from build123d import *

# Parameters (mm, degrees)
SKETCH2_W                     = 6.6
SKETCH2_H                     = 9.76
BOSS_EXTRUDE1_DEPTH           = 1.75
BOSS_EXTRUDE1_TAPER           = 15
BOSS_EXTRUDE1_OTHER_WAY_DEPTH = 1.75
BOSS_EXTRUDE1_OTHER_WAY_TAPER = 15
BOSS_EXTRUDE2_DEPTH           = 0.65
FILLET1_R                     = 0.15
BOSS_EXTRUDE3_DEPTH           = 0.65
BOSS_EXTRUDE4_DEPTH           = 0.65
BOSS_EXTRUDE5_DEPTH           = 0.65


with BuildPart() as part:
    # Sketch2 → Boss-Extrude1 (new body)
    with BuildSketch(Plane(origin=(0, 0, 0), x_dir=(1, 0, 0), z_dir=(0, 1, 0))):
        Rectangle(SKETCH2_W, SKETCH2_H)
    extrude(amount=BOSS_EXTRUDE1_DEPTH, taper=BOSS_EXTRUDE1_TAPER)

    # Sketch2 → Boss-Extrude1 other way (add)
    with BuildSketch(Plane(origin=(0, 0, 0), x_dir=(1, 0, 0), z_dir=(0, 1, 0))):
        Rectangle(SKETCH2_W, SKETCH2_H)
    extrude(amount=-BOSS_EXTRUDE1_OTHER_WAY_DEPTH, taper=BOSS_EXTRUDE1_OTHER_WAY_TAPER)

    # Sketch3 → Boss-Extrude2 (add, symmetric)
    with BuildSketch(Plane.XY.offset(3.66)):
        Polygon((3.266506351, 0.125), (3.3, 0), (3.266506351, -0.125), (3.616889449, -0.125), (4.25, -2.55), (5.15, -2.55), (5.15, -2.3), (4.443110551, -2.3), (3.81, 0.125), align=None)
        Polygon((-4.25, -2.55), (-5.15, -2.55), (-5.15, -2.3), (-4.443110551, -2.3), (-3.81, 0.125), (-3.266506351, 0.125), (-3.3, 0), (-3.266506351, -0.125), (-3.616889449, -0.125), align=None)
    extrude(amount=BOSS_EXTRUDE2_DEPTH, both=True)

    # Fillet1
    fillet1_edges = [part.edges().sort_by_distance(p)[0] for p in [
        (4.443110551, -2.3, 3.66),
        (3.81, 0.125, 3.66),
        (3.616889449, -0.125, 3.66),
        (4.25, -2.55, 3.66),
        (-4.25, -2.55, 3.66),
        (-3.616889449, -0.125, 3.66),
        (-3.81, 0.125, 3.66),
        (-4.443110551, -2.3, 3.66),
    ]]
    fillet(fillet1_edges, radius=FILLET1_R)

    # Sketch5 → Boss-Extrude3 (add, symmetric)
    with BuildSketch(Plane.XY.offset(1.22)):
        with BuildLine():
            Line((-5.15, -2.55), (-4.365866331, -2.55))
            ThreePointArc((-4.365866331, -2.55), (-4.274170395, -2.518709121), (-4.220731079, -2.437891406))
            Line((-4.220731079, -2.437891406), (-3.64615837, -0.237108594))
            ThreePointArc((-3.64615837, -0.237108594), (-3.592719053, -0.156290879), (-3.501023118, -0.125))
            Line((-3.501023118, -0.125), (-3.266506351, -0.125))
            Line((-3.266506351, -0.125), (-3.3, 0))
            Line((-3.3, 0), (-3.266506351, 0.125))
            Line((-3.266506351, 0.125), (-3.694133669, 0.125))
            ThreePointArc((-3.694133669, 0.125), (-3.785829605, 0.093709121), (-3.839268921, 0.012891406))
            Line((-3.839268921, 0.012891406), (-4.41384163, -2.187891406))
            ThreePointArc((-4.41384163, -2.187891406), (-4.467280947, -2.268709121), (-4.558976882, -2.3))
            Line((-4.558976882, -2.3), (-5.15, -2.3))
            Line((-5.15, -2.3), (-5.15, -2.55))
        make_face()
        with BuildLine():
            Line((3.64615837, -0.237108594), (4.220731079, -2.437891406))
            ThreePointArc((4.220731079, -2.437891406), (4.274170395, -2.518709121), (4.365866331, -2.55))
            Line((4.365866331, -2.55), (5.15, -2.55))
            Line((5.15, -2.55), (5.15, -2.3))
            Line((5.15, -2.3), (4.558976882, -2.3))
            ThreePointArc((4.558976882, -2.3), (4.467280947, -2.268709121), (4.41384163, -2.187891406))
            Line((4.41384163, -2.187891406), (3.839268921, 0.012891406))
            ThreePointArc((3.839268921, 0.012891406), (3.785829605, 0.093709121), (3.694133669, 0.125))
            Line((3.694133669, 0.125), (3.266506351, 0.125))
            Line((3.266506351, 0.125), (3.3, 0))
            Line((3.3, 0), (3.266506351, -0.125))
            Line((3.266506351, -0.125), (3.501023118, -0.125))
            ThreePointArc((3.501023118, -0.125), (3.592719053, -0.156290879), (3.64615837, -0.237108594))
        make_face()
    extrude(amount=BOSS_EXTRUDE3_DEPTH, both=True)

    # Sketch6 → Boss-Extrude4 (add, symmetric)
    with BuildSketch(Plane.XY.offset(-1.22)):
        with BuildLine():
            Line((3.64615837, -0.237108594), (4.220731079, -2.437891406))
            ThreePointArc((4.220731079, -2.437891406), (4.274170395, -2.518709121), (4.365866331, -2.55))
            Line((4.365866331, -2.55), (5.15, -2.55))
            Line((5.15, -2.55), (5.15, -2.3))
            Line((5.15, -2.3), (4.558976882, -2.3))
            ThreePointArc((4.558976882, -2.3), (4.467280947, -2.268709121), (4.41384163, -2.187891406))
            Line((4.41384163, -2.187891406), (3.839268921, 0.012891406))
            ThreePointArc((3.839268921, 0.012891406), (3.785829605, 0.093709121), (3.694133669, 0.125))
            Line((3.694133669, 0.125), (3.266506351, 0.125))
            Line((3.266506351, 0.125), (3.3, 0))
            Line((3.3, 0), (3.266506351, -0.125))
            Line((3.266506351, -0.125), (3.501023118, -0.125))
            ThreePointArc((3.501023118, -0.125), (3.592719053, -0.156290879), (3.64615837, -0.237108594))
        make_face()
        with BuildLine():
            Line((-5.15, -2.55), (-4.365866331, -2.55))
            ThreePointArc((-4.365866331, -2.55), (-4.274170395, -2.518709121), (-4.220731079, -2.437891406))
            Line((-4.220731079, -2.437891406), (-3.64615837, -0.237108594))
            ThreePointArc((-3.64615837, -0.237108594), (-3.592719053, -0.156290879), (-3.501023118, -0.125))
            Line((-3.501023118, -0.125), (-3.266506351, -0.125))
            Line((-3.266506351, -0.125), (-3.3, 0))
            Line((-3.3, 0), (-3.266506351, 0.125))
            Line((-3.266506351, 0.125), (-3.694133669, 0.125))
            ThreePointArc((-3.694133669, 0.125), (-3.785829605, 0.093709121), (-3.839268921, 0.012891406))
            Line((-3.839268921, 0.012891406), (-4.41384163, -2.187891406))
            ThreePointArc((-4.41384163, -2.187891406), (-4.467280947, -2.268709121), (-4.558976882, -2.3))
            Line((-4.558976882, -2.3), (-5.15, -2.3))
            Line((-5.15, -2.3), (-5.15, -2.55))
        make_face()
    extrude(amount=BOSS_EXTRUDE4_DEPTH, both=True)

    # Sketch7 → Boss-Extrude5 (add, symmetric)
    with BuildSketch(Plane.XY.offset(-3.66)):
        with BuildLine():
            Line((3.64615837, -0.237108594), (4.220731079, -2.437891406))
            ThreePointArc((4.220731079, -2.437891406), (4.274170395, -2.518709121), (4.365866331, -2.55))
            Line((4.365866331, -2.55), (5.15, -2.55))
            Line((5.15, -2.55), (5.15, -2.3))
            Line((5.15, -2.3), (4.558976882, -2.3))
            ThreePointArc((4.558976882, -2.3), (4.467280947, -2.268709121), (4.41384163, -2.187891406))
            Line((4.41384163, -2.187891406), (3.839268921, 0.012891406))
            ThreePointArc((3.839268921, 0.012891406), (3.785829605, 0.093709121), (3.694133669, 0.125))
            Line((3.694133669, 0.125), (3.266506351, 0.125))
            Line((3.266506351, 0.125), (3.3, 0))
            Line((3.3, 0), (3.266506351, -0.125))
            Line((3.266506351, -0.125), (3.501023118, -0.125))
            ThreePointArc((3.501023118, -0.125), (3.592719053, -0.156290879), (3.64615837, -0.237108594))
        make_face()
        with BuildLine():
            Line((-5.15, -2.3), (-5.15, -2.55))
            Line((-5.15, -2.55), (-4.365866331, -2.55))
            ThreePointArc((-4.365866331, -2.55), (-4.274170395, -2.518709121), (-4.220731079, -2.437891406))
            Line((-4.220731079, -2.437891406), (-3.64615837, -0.237108594))
            ThreePointArc((-3.64615837, -0.237108594), (-3.592719053, -0.156290879), (-3.501023118, -0.125))
            Line((-3.501023118, -0.125), (-3.266506351, -0.125))
            Line((-3.266506351, -0.125), (-3.3, 0))
            Line((-3.3, 0), (-3.266506351, 0.125))
            Line((-3.266506351, 0.125), (-3.694133669, 0.125))
            ThreePointArc((-3.694133669, 0.125), (-3.785829605, 0.093709121), (-3.839268921, 0.012891406))
            Line((-3.839268921, 0.012891406), (-4.41384163, -2.187891406))
            ThreePointArc((-4.41384163, -2.187891406), (-4.467280947, -2.268709121), (-4.558976882, -2.3))
            Line((-4.558976882, -2.3), (-5.15, -2.3))
        make_face()
    extrude(amount=BOSS_EXTRUDE5_DEPTH, both=True)


solid = part.part
Input: part model. Units: mm. Frame: model coordinates. A direction names the side the tool comes from. Round coordinates to 2 decimals unless told otherwise and drop trailing zeros.
1) Draft query along X for faces 1 (the flat face through (0, 1.75, 0)), 2 (the flat face through (3.93, -1.32, -1.23)), 3 (the flat face through (4.13, -1.1, -1.23)). Return one class per face: pulls with the +X half, pulls with the -X half, needs draft (parallel to the pull), parting line crosses it, or undercut.
2) Contact query for flat-ended pins moving along their axis: P1, Ø2, axis at y = -2, z = 1.5, coming from the -X side; P2, Ø0.7, axis at x = -5, z = 3.5, coming from the +Y side; P3, Ø2, axis at x = 4, y = -1, coming from the -Z side; P4, Ø2, axis at x = 4.5, y = -2, coming from the -Z side. Output: stop coordinate, or through.
3) Reachability of faces 4 (the flat face through (3.93, -1.32, -3.67)), 5 (the flat face through (4.13, -1.1, 1.23)) from +Z, -Z, +X, -X, +Y, -Y: full face, straight path, thin tool, end or side. Return the list, or none.
4) Cut plane A-A (y = -1.15). Count the separate pieces of the cut face and the enclosed holes in it, then the cut area to 3 significant figures.
5) Ray query, L1, parallel to Z at x = -4.25, y = -2.25; L2, parallel to X at y = -1.15, z = -3.25; L3, parallel to Y at x = 2.25, z = 4. Return the intervals inside material, ascending.
Geometry says:
1. face 1: needs draft
1. face 2: undercut
1. face 3: pulls with the +X half
2. P1: stops at x = -5.15
2. P2: stops at y = -2.3
2. P3: stops at z = -4.77
2. P4: stops at z = -4.31
3. face 4: +Z, -Z, -Y
3. face 5: +Z, -Z, +X, +Y
4. separate pieces: 9
4. enclosed holes: 0
4. area: 57.4 mm2
5. L1: z = -4.31 to -3.01, -1.87 to -0.57, 0.57 to 1.87, 3.01 to 4.31
5. L2: x = -4.14 to -3.88, -2.99 to 2.99, 3.88 to 4.14
5. L3: y = -1.75 to 1.75
